```python
from build123d import *

# Parameters (mm, degrees)
F0_R     = 38.1
F0_R_2   = 19.1135
F1_DEPTH = 6.35
F4_D     = 4.0386
F7_D     = 4.0386


with BuildPart() as f1:
    # F0 (on Front) → F1 (new body)
    with BuildSketch(Plane.XZ):
        Circle(F0_R)
        Circle(F0_R_2, mode=Mode.SUBTRACT)
    extrude(amount=F1_DEPTH)

    # F4 (through all)
    with Locations(Plane.XY.offset(38.1)):
        with Locations((0, -3.175)):
            Hole(F4_D / 2)

    # F7 (through all)
    with Locations(Plane.YZ.offset(38.1)):
        with Locations((-3.175, 0)):
            Hole(F7_D / 2)


solid = f1.part
```
Geometry: final body of the model. Coordinates: model frame, mm. Give positions to 0.01 mm unless a question says otherwise; leave off trailing zeros. Order: outer loops, then holes, each group sorted by start corner. A loop starts at its lowest first (then second) coordinate and runs counter-clockwise, first axis right, second up. Notation, with made-up numbers: M 28.25,-15 L 70.25,-15 A21 cw 70.25,-10 Z; hole C 19.25,-40 d8. An arc over 180 degrees is marked long. Answer as CSV lines item,"result". Start each with the question number.
1) Cut plane C-C (z = 15). Output: boundary loops of the cut face in (x, y), then the cut area to 3 significant figures.
2) First-contact query: P1, Ø2, axis at x = 2, y = -3.5, coming from the -Z side; P2, Ø3, axis at x = 0, y = -3.175, coming from the -Z side; P3, Ø8, axis at x = -27.5, z = -1.5, coming from the +Y side; P4, Ø1, axis at x = -28.5, y = -4.5, coming from the -Z side. Flat tips, straight axial feed; report the tip coordinate or a pass-through.
3) Line query: line 1 (Y direction, x = 0, z = -29); line 2 (Z direction, x = 22, y = -4.5); line 3 (X direction, y = -4, z = -20.5). Output: solid intervals per line, ascending. Write a range as from..to.
4) Mould query, pull axis X, two halves, no side actions, for faces 1 (the cylindrical face through (-28.69, -5.1, 0.61)), 2 (the cylindrical face through (36.34, -3.13, 11.44)), 3 (the cylindrical face through (18.23, -3.13, 5.74)). Classes: +X half, -X half, draft (parallel to the pull), parting line (faces both ways), or undercut.
5) Cut plane A-A (x = 0). Output: boundary loops of the cut face in (y, z).
6) Cut plane B-B (z = 0). Output: boundary loops of the cut face in (x, y).
7) Cut plane D-D (x = 25). Output: boundary loops of the cut face in (y, z) (3 decimals), then the cut area to 3 significant figures.
Findings below:
1,outline,"M -35.02,-6.35 L -11.85,-6.35 L -11.85,0 L -35.02,0 Z; M 11.85,-6.35 L 35.02,-6.35 L 35.02,0 L 11.85,0 Z"
1,area,"294 mm²"
2,P1,"stops at z = -38.07"
2,P2,"passes through"
2,P3,"stops at y = 0"
2,P4,"stops at z = -25.84"
3,line 1,"y = -6.35..-5.19, -1.16..0"
3,line 2,"z = -31.11..-1.52, 1.52..31.11"
3,line 3,"x = -32.11..-1.84, 1.84..32.11"
4,face 1,"draft"
4,face 2,"parting line"
4,face 3,"undercut"
5,outline,"M -6.35,-38.1 L -5.19,-38.1 L -5.19,-19.11 L -6.35,-19.11 Z; M -6.35,19.11 L -5.19,19.11 L -5.19,38.1 L -6.35,38.1 Z; M -1.16,-38.1 L 0,-38.1 L 0,-19.11 L -1.16,-19.11 Z; M -1.16,19.11 L 0,19.11 L 0,38.1 L -1.16,38.1 Z"
6,outline,"M -38.1,-6.35 L -19.11,-6.35 L -19.11,-5.19 L -38.1,-5.19 Z; M -38.1,-1.16 L -19.11,-1.16 L -19.11,0 L -38.1,0 Z; M 19.11,-6.35 L 38.1,-6.35 L 38.1,-5.19 L 19.11,-5.19 Z; M 19.11,-1.16 L 38.1,-1.16 L 38.1,0 L 19.11,0 Z"
7,outline,"M -6.35,-28.751 L 0,-28.751 L 0,28.751 L -6.35,28.751 Z; hole C -3.175,0 d4.039"
7,area,"352 mm²"
